Design review of the part built by this model. Coordinates are the model's own, in mm. A direction names the side the tool comes from. Coordinates: 2 decimals unless noted, no trailing zeros. Write each loop counter-clockwise with the first axis right and the second up, starting at its lowest first coordinate (ties: lowest second). Pieces come first, ordered by that corner, then holes.
Q1. Take a section at C-C (x = -10). Give the boundary of the cut face in (y, z).
Q2. Take a section at A-A (z = 15). Give the boundary of the cut face in (x, y), and give its area (3 significant figures).
Q3. Take a section at B-B (y = 12). Give the boundary of the cut face in (x, z).
Q4. Take a section at D-D (z = 10). Give the boundary of the cut face in (x, y).
Q5. Machinability: for faces 4 (the cylindrical face through (-70, 30, 6)), 5 (the flat face through (-11.5, 30, 17)), which of the approach directions +Z, -Z, +X, -X, +Y, -Y give a long, thin tool a straight path to every point of the face, cutting with its end or side? Answer none if there is none.
Q6. Mouldability with a two-part tool opening along X and no side actions: class faces 1 (the flat face through (-76, 30, 20)), 2 (the flat face through (-8.5, 30, 17)), 3 (the flat face through (0, 30, 10)) as pulls with the +X half, pulls with the -X half, needs draft (parallel to the pull), parting line crosses it, or undercut.
Q7. Insertion check: pin 1 (6.5 mm diameter, centred on x = -10, z = 10, fed in from -Y). The pin has a flat end and moves straight along its axis. Give the tip position at first contact, or say it passes through.
Q8. For probe 1 along X at (y, z) = (29, 14); probe 2 along X at (y, z) = (23, 10); probe 3 along Z at (x, y) = (-68, 27.5), list the stretches that pass through material, from the lowest coordinate up.
Autodesk Inventor part; units mm, degrees
ref_plane "YZ Plane" through (0, 0, 0) normal (1, 0, 0) x (0, 1, 0)
ref_plane "XZ Plane" through (0, 0, 0) normal (0, 1, 0) x (-1, 0, 0)
ref_plane "XY Plane" through (0, 0, 0) normal (0, 0, 1) x (1, 0, 0)
sketch "Sketch1" plane through (0, 0, 0) normal (0, 1, 0) x (-1, 0, 0)
  arc A0 (8.5, 13.7081) -> (11.5, 13.7081) centre (10, 10) ccw
  line L0 (8.5, 20) -> (8.5, 13.7081)
  line L1 (11.5, 20) -> (11.5, 13.7081)
  line L2 (10, 20) -> (10, 18.7339)
  line L3 (20, 20) -> (10, 20)
  line L4 (8.5, 20) -> (0, 20)
  line L5 (0, 20) -> (0, 0)
  line L6 (0, 0) -> (20, 0)
  line L7 (20, 0) -> (20, 20)
  arc A1 (68.5, 13.7081) -> (71.5, 13.7081) centre (70, 10) ccw
  line L8 (68.5, 20) -> (68.5, 13.7081)
  line L9 (71.5, 20) -> (71.5, 13.7081)
  line L10 (70, 20) -> (70, 18.3732)
  line L11 (80, 20) -> (70, 20)
  line L12 (68.5, 20) -> (60.9559, 20)
  line L13 (60.9559, 20) -> (60.9559, 0)
  line L14 (60.9559, 0) -> (80, 0)
  line L15 (80, 0) -> (80, 20)
  line L16 (60.9559, 0) -> (20, 0)
  line L17 (20, 0) -> (20, 20)
  line L18 (20, 20) -> (60.9559, 20)
  line L19 (60.9559, 20) -> (60.9559, 0)
  dimension "d2" = 8
  dimension "d7" = 1.5
  dimension "d8" = 1.5
  dimension "d16" = 10
  dimension "d17" = 8
  dimension "d18" = 1.5
  dimension "d19" = 1.5
  dimension "d20" = 10
  dimension "d22" = 80
  dimension "d23" = 10
  dimension "d24" = 0
  dimension "d25" = 60
  dimension "d26" = 20
  dimension "d27" = 20
  dimension "d28" = 20
  dimension "d29" = 20
  dimension "d30" = 10
  dimension "d31" = 10
  dimension "d32" = 20
extrude "Extrusion1" add sketch "Sketch1" along normal blind 60
equation "\"d2\" = RodDiameter"
equation "\"d17\" = d2"
equation "\"RodDiameter\" = 8"
equation "\"VerticalBearingOD\" = 16"
equation "\"PrintingClearance\" = 0.2"
equation "\"d21\" = 8"
properties part number "GantryHolder"
Response:
1. outline: (0, 0) - (60, 0) - (60, 6) - (0, 6) - close
2. outline: (-80, 0) - (-71.5, 0) - (-71.5, 60) - (-80, 60) - close; (-68.5, 0) - (-11.5, 0) - (-11.5, 60) - (-68.5, 60) - close; (-8.5, 0) - (0, 0) - (0, 60) - (-8.5, 60) - close
2. area: 4,440 mm2
3. outline: (-80, 0) - (0, 0) - (0, 20) - (-8.5, 20) - (-8.5, 13.71) arc R4 cw (long way) to (-11.5, 13.71) - (-11.5, 20) - (-68.5, 20) - (-68.5, 13.71) arc R4 cw (long way) to (-71.5, 13.71) - (-71.5, 20) - (-80, 20) - close
4. outline: (-80, 0) - (-74, 0) - (-74, 60) - (-80, 60) - close; (-66, 0) - (-14, 0) - (-14, 60) - (-66, 60) - close; (-6, 0) - (0, 0) - (0, 60) - (-6, 60) - close
5. face 4: +Y, -Y
5. face 5: +Z, +Y, -Y
6. face 1: needs draft
6. face 2: undercut
6. face 3: pulls with the +X half
7. pin 1: passes through
8. probe 1: x = -80 to -71.5, -68.5 to -11.5, -8.5 to 0
8. probe 2: x = -80 to -74, -66 to -14, -6 to 0
8. probe 3: z = 0 to 6.54, 13.46 to 20
